Input: dimensioned drawing with shaded views. Units: mm. Origin: part minimum x, y, z. Coordinates: 2 decimals unless noted, no trailing zeros. Order: outer loops, then holes, each group sorted by start corner. A loop starts at its lowest first (then second) coordinate and runs counter-clockwise, first axis right, second up. Notation, with made-up numbers: M -28.5,-3.75 L 18.5,-3.75 A17 cw 18.5,8.25 Z; hole C -7,-17 d10. An arc over 180 degrees is marked long. Write item = value, one per line.
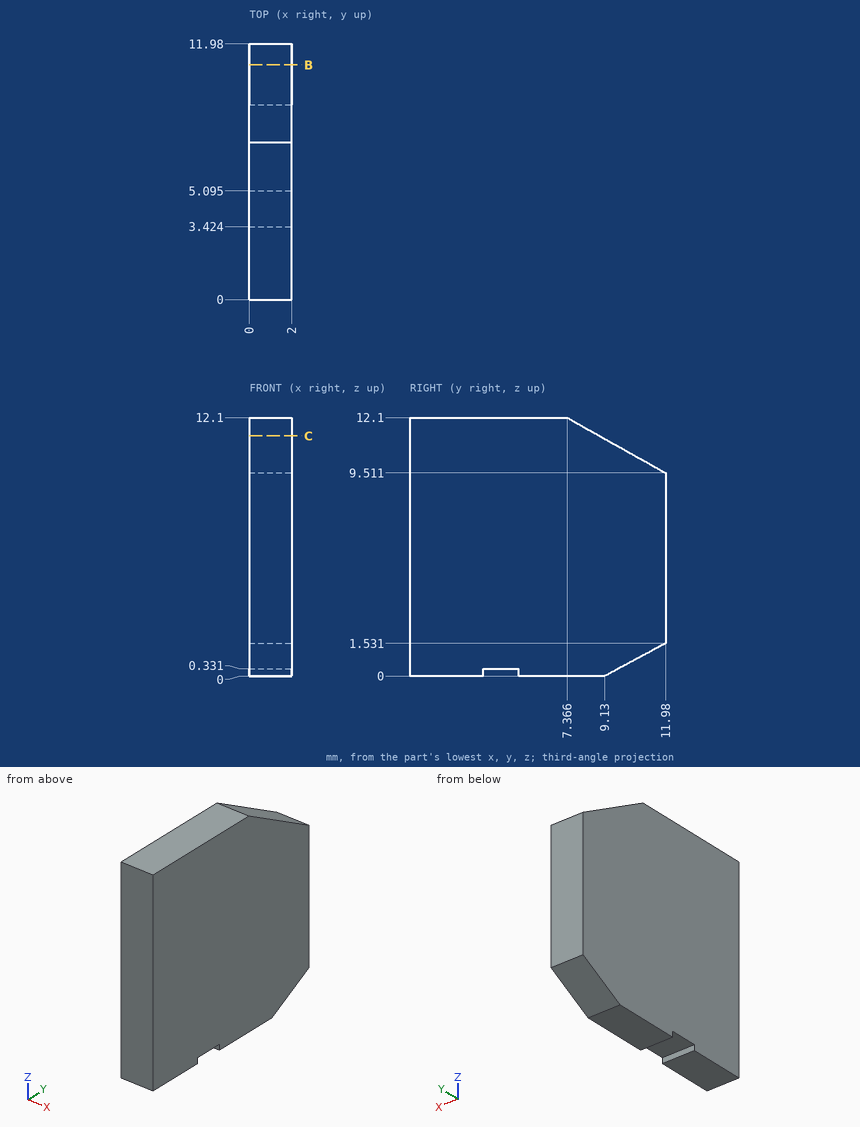
1) Section C-C, the plane z = 11.25. Return loops of the section in (x, y).
Numbers:
outline = M 0,0 L 2,0 L 2,8.88 L 0,8.88 Z
2) Line query: L1, parallel to Z at x = 0.6, y = 3.75; L2, parallel to Z at x = 0.85, y = 9.75 (1 decimal); L3, parallel to Y at x = 1.6, z = 11.5 (1 decimal). Output: solid intervals per line, ascending.
Numbers:
L1 = 0.33 to 12.1
L2 = 0.3 to 10.8
L3 = 0 to 8.4
3) Section B-B, the plane y = 11. Return loops of the section in (x, z) (1 decimal).
Numbers:
outline = M 0,1 L 2,1 L 2,10.1 L 0,10.1 Z
